Source: CAD feature listing. Evaluate the final solid. Frame: model axes, mm. Face numbers are marked on the shaded views. Round coordinates to 2 decimals unless told otherwise and drop trailing zeros. Loops run counter-clockwise (first coordinate to the right, second up) from the corner with the lowest first, then second, coordinate; pieces in that order, holes last. Notation, with made-up numbers: (-23.5, 42.25) - (-11.5, 42.25) arc R24 cw to (-11.5, 78.25) - close; hole circle Ø4 at (84.25, 2.25). An arc over 180 degrees is marked (long way). One line per question, with ' | ' between items.
Autodesk Inventor part; units mm, degrees
ref_plane "YZ Plane" through (0, 0, 0) normal (1, 0, 0) x (0, 1, 0)
ref_plane "XZ Plane" through (0, 0, 0) normal (0, 1, 0) x (-1, 0, 0)
ref_plane "XY Plane" through (0, 0, 0) normal (0, 0, 1) x (1, 0, 0)
sketch "Boceto1" plane through (0, 0, 0) normal (0, 0, 1) x (1, 0, 0)
  line L0 (-198, 0) -> (0, 0)
  line L1 (-198, 0) -> (-198, -2)
  line L2 (0, -2) -> (-198, -2)
  line L3 (0, 0) -> (0, -2)
  line L4 (0, -2) -> (0, -200)
  line L5 (0, -2) -> (-2, -2)
  line L6 (-2, -200) -> (-2, -2)
  line L7 (0, -200) -> (-2, -200)
  line L8 (-2, -200) -> (-200, -200)
  line L9 (-2, -200) -> (-2, -198)
  line L10 (-200, -198) -> (-2, -198)
  line L11 (-200, -200) -> (-200, -198)
  line L12 (-200, -198) -> (-200, 0)
  line L13 (-200, -198) -> (-198, -198)
  line L14 (-198, 0) -> (-198, -198)
  line L15 (-200, 0) -> (-198, 0)
  line L16 (0, 0) -> (0, 1.6)
  line L17 (0, 1.6) -> (1.6, 1.6)
  line L18 (1.6, 1.6) -> (-201.6, 1.6)
  line L19 (-201.6, 1.6) -> (-201.6, -201.6)
  line L20 (-201.6, -201.6) -> (1.6, -201.6)
  line L21 (1.6, -201.6) -> (1.6, 1.6)
  line L22 (-203, 1) -> (-203, -201)
  line L23 (-201, -203) -> (1, -203)
  line L24 (3, -201) -> (3, 1)
  line L25 (1, 3) -> (-201, 3)
  line L26 (-192.75, -7.25) -> (-7.25, -7.25)
  line L27 (-7.25, -7.25) -> (-7.25, -192.75)
  line L28 (-7.25, -192.75) -> (-192.75, -192.75)
  line L29 (-192.75, -192.75) -> (-192.75, -7.25)
  circle A0 centre (-195.25, -4.75) radius 2.1
  circle A1 centre (-4.75, -4.75) radius 2.1
  circle A2 centre (-4.75, -195.25) radius 2.1
  circle A3 centre (-195.25, -195.25) radius 2.1
  arc A4 (-201, 3) -> (-203, 1) centre (-201, 1) ccw
  arc A5 (-203, -201) -> (-201, -203) centre (-201, -201) ccw
  arc A6 (1, -203) -> (3, -201) centre (1, -201) ccw
  arc A7 (3, 1) -> (1, 3) centre (1, 1) ccw
  dimension "d0" = 1.6
  dimension "d1" = 1.6
  dimension "d2" = 203.2
  dimension "d3" = 203.2
extrude "Extrusión1" add sketch "Boceto1" along normal blind 1.2 contours L17 L21 L20 L19 L18 | L0 L3 L2 L1 | L1 L14 L10 L12 L15 | L2 L6 L10 L14 | L4 L7 L6 L2 | L10 L6 L8 L11 | A4 L25 A7 L24 A6 L23 A5 L22 | L26 L27 L28 L29 | A0 | A1 | A2 | A3
sketch "Boceto2" plane through (0, 0, 1.2) normal (0, 0, 1) x (1, 0, 0)
  line L0 (-192.75, -7.25) -> (-7.25, -7.25)
  line L1 (-7.25, -7.25) -> (-7.25, -192.75)
  line L2 (-2.25, -197.75) -> (-2.25, -2.25)
  line L3 (-2.25, -2.25) -> (-197.75, -2.25)
  line L4 (-7.25, -7.25) -> (-2.25, -2.25)
  circle A0 centre (-4.75, -4.75) radius 1.5
  line L5 (-201, -203) -> (1, -203)
  line L6 (-203, -203) -> (-203, -195.25)
  line L7 (-203, 1) -> (-203, -201)
  line L8 (-203, -195.25) -> (-195.25, -195.25)
  circle A1 centre (-195.25, -195.25) radius 1.5
  line L9 (3, -203) -> (-4.75, -203)
  line L10 (-4.75, -203) -> (-4.75, -195.25)
  circle A2 centre (-4.75, -195.25) radius 1.5
  line L11 (-203, 3) -> (-195.25, 3)
  line L12 (1, 3) -> (-201, 3)
  line L13 (-195.25, 3) -> (-195.25, -4.75)
  circle A3 centre (-195.25, -4.75) radius 1.5
  point P0 (0, 0)
  point P1 (3, 3)
  dimension "d6" = 3
  dimension "d14" = 7.75
  dimension "d15" = 7.75
  dimension "d16" = 3
  dimension "d17" = 7.75
  dimension "d18" = 7.75
  dimension "d19" = 3
  dimension "d20" = 7.75
  dimension "d21" = 7.75
  dimension "d22" = 90
  dimension "d23" = 3
hole "Agujero1" at (-4.75, -4.75, 1.2) at (-195.25, -4.75, 1.2) at (-195.25, -195.25, 1.2) at (-4.75, -195.25, 1.2) direction (0, 0, -1) diameter 3 depth 4
sketch "Boceto3" plane through (0, 0, 1.2) normal (0, 0, 1) x (1, 0, 0)
  line L0 (-125, -122.5) -> (-75, -122.5)
  arc A0 (-75, -122.5) -> (-70, -117.5) centre (-75, -117.5) ccw
  line L1 (-70, -117.5) -> (-70, -112.2474)
  arc A1 (-64, -104.899) -> (-70, -112.2474) centre (-62.5, -112.2474) ccw
  arc A2 (-64, -104.899) -> (-64, -95.101) centre (-65, -100) ccw
  arc A3 (-70, -87.7526) -> (-64, -95.101) centre (-62.5, -87.7526) ccw
  line L2 (-70, -87.7526) -> (-70, -82.5)
  arc A4 (-70, -82.5) -> (-75, -77.5) centre (-75, -82.5) ccw
  line L3 (-75, -77.5) -> (-125, -77.5)
  arc A5 (-125, -77.5) -> (-130, -82.5) centre (-125, -82.5) ccw
  line L4 (-130, -82.5) -> (-130, -87.7526)
  arc A6 (-136, -95.101) -> (-130, -87.7526) centre (-137.5, -87.7526) ccw
  arc A7 (-136, -95.101) -> (-136, -104.899) centre (-135, -100) ccw
  arc A8 (-130, -112.2474) -> (-136, -104.899) centre (-137.5, -112.2474) ccw
  line L5 (-130, -112.2474) -> (-130, -117.5)
  arc A9 (-130, -117.5) -> (-125, -122.5) centre (-125, -117.5) ccw
  line L6 (-125, -121.5) -> (-75, -121.5)
  arc A10 (-75, -121.5) -> (-71, -117.5) centre (-75, -117.5) ccw
  line L7 (-71, -117.5) -> (-71, -82.5)
  arc A11 (-71, -82.5) -> (-75, -78.5) centre (-75, -82.5) ccw
  line L8 (-75, -78.5) -> (-125, -78.5)
  arc A12 (-125, -78.5) -> (-129, -82.5) centre (-125, -82.5) ccw
  line L9 (-129, -82.5) -> (-129, -117.5)
  arc A13 (-129, -117.5) -> (-125, -121.5) centre (-125, -117.5) ccw
  line L10 (-75, -118) -> (-125, -118)
  arc A14 (-125.5, -117.5) -> (-125, -118) centre (-125, -117.5) ccw
  line L11 (-125.5, -117.5) -> (-125.5, -82.5)
  arc A15 (-125, -82) -> (-125.5, -82.5) centre (-125, -82.5) ccw
  line L12 (-125, -82) -> (-75, -82)
  arc A16 (-74.5, -82.5) -> (-75, -82) centre (-75, -82.5) ccw
  line L13 (-74.5, -82.5) -> (-74.5, -117.5)
  arc A17 (-75, -118) -> (-74.5, -117.5) centre (-75, -117.5) ccw
  line L14 (-74.5, -118) -> (-74.5, -82)
  line L15 (-78, -118) -> (-78, -82)
  line L16 (-81, -118) -> (-81, -82)
  line L17 (-88, -118) -> (-88, -82)
  line L18 (-91, -118) -> (-91, -82)
  line L19 (-98, -118) -> (-98, -82)
  line L20 (-101, -118) -> (-101, -82)
  line L21 (-108, -118) -> (-108, -82)
  line L22 (-111, -118) -> (-111, -82)
  line L23 (-118, -118) -> (-118, -82)
  line L24 (-121, -118) -> (-121, -82)
  circle A18 centre (-65, -100) radius 1.5
  circle A19 centre (-135, -100) radius 1.5
  point P0 (0, 0)
  dimension "d24" = 3.5
  dimension "d25" = 3
  dimension "d26" = 7
  dimension "d27" = 3
  dimension "d28" = 7
  dimension "d29" = 3
  dimension "d30" = 7
  dimension "d31" = 3
  dimension "d32" = 7
  dimension "d33" = 3
  dimension "d36" = 3
  dimension "d37" = 3
extrude "Extrusión2" cut sketch "Boceto3" against normal blind 3 contours L10 L16 L12 L15 | L10 L18 L12 L17 | L10 L20 L12 L19 | L10 L22 L12 L21 | L10 L24 L12 L23 | A18 | A19
properties part number "Tapadera"
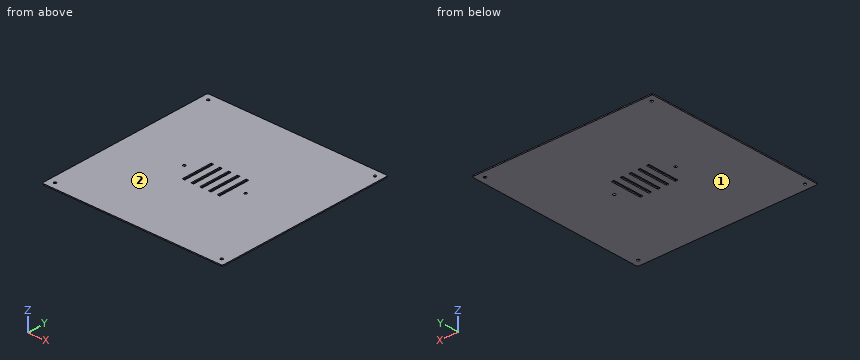
1. Section query A-A, the plane y = -115. Return loops of the section in (x, z).
Worked out:
outline: (-203, 0) - (-121, 0) - (-121, 1.2) - (-203, 1.2) - close; (-118, 0) - (-111, 0) - (-111, 1.2) - (-118, 1.2) - close; (-108, 0) - (-101, 0) - (-101, 1.2) - (-108, 1.2) - close; (-98, 0) - (-91, 0) - (-91, 1.2) - (-98, 1.2) - close; (-88, 0) - (-81, 0) - (-81, 1.2) - (-88, 1.2) - close; (-78, 0) - (3, 0) - (3, 1.2) - (-78, 1.2) - close
2. Material intervals for probe 1 along X at (y, z) = (-195.25, 0.65); probe 2 along X at (y, z) = (-89, 0.35), sorted ascending.
Worked out:
probe 1: x = -203 to -196.75, -193.75 to -6.25, -3.25 to 3 | probe 2: x = -203 to -121, -118 to -111, -108 to -101, -98 to -91, -88 to -81, -78 to 3
3. Contact query for a flat-ended pin moving along its axis: P1, Ø1.8, axis at x = -195.25, y = -4.75, coming from the +Z side. Output: stop coordinate, or through.
Worked out:
P1: passes through
4. Mould query, pull axis Z, two halves, no side actions, for the marked faces 1 and 2. Classes: released by +Z, released by -Z, zero draft, split by the parting line, or undercut.
Worked out:
face 1: released by -Z | face 2: released by +Z
